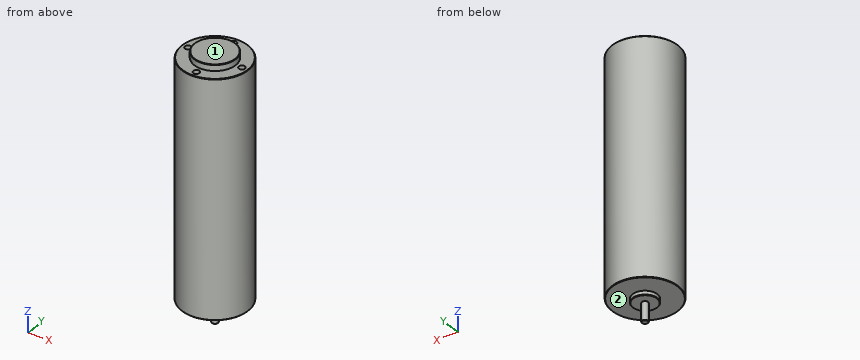
from build123d import *

# Parameters (mm, degrees)
CROQUIS1_R              = 16
SALIENTE_EXTRUIR1_DEPTH = 113.4
CROQUIS2_R              = 10
SALIENTE_EXTRUIR2_DEPTH = 3
CROQUIS3_R              = 6
SALIENTE_EXTRUIR3_DEPTH = 2
CROQUIS4_R              = 1.5
SALIENTE_EXTRUIR4_DEPTH = 9
CHAFL_N1_SIZE           = 0.2
CROQUIS5_R              = 1.5
CORTAR_EXTRUIR1_DEPTH   = 4


with BuildPart() as part:
    # Croquis1 → Saliente-Extruir1 (new body)
    with BuildSketch(Plane.XY):
        with Locations(Location((0, 0, 0), (0, 0, 180))):
            Circle(CROQUIS1_R)
    extrude(amount=SALIENTE_EXTRUIR1_DEPTH)

    # Croquis2 → Saliente-Extruir2 (add)
    with BuildSketch(Plane.XY.offset(113.4)):
        Circle(CROQUIS2_R)
    extrude(amount=SALIENTE_EXTRUIR2_DEPTH)

    # Croquis3 → Saliente-Extruir3 (add)
    with BuildSketch(Plane(origin=(0, 0, 0), x_dir=(-1, 0, 0), z_dir=(0, 0, -1))):
        Circle(CROQUIS3_R)
    extrude(amount=SALIENTE_EXTRUIR3_DEPTH)

    # Croquis4 → Saliente-Extruir4 (add)
    with BuildSketch(Plane(origin=(0, 0, -2), x_dir=(-1, 0, 0), z_dir=(0, 0, -1))):
        Circle(CROQUIS4_R)
    extrude(amount=SALIENTE_EXTRUIR4_DEPTH)

    # Chaflán1
    chafl_n1_edges = [part.edges().sort_by_distance(p)[0] for p in [
        (6, 0, -2),
        (1.5, 0, -11),
        (16, 0, 0),
        (16, 0, 113.4),
        (-10, 0, 116.4),
    ]]
    chamfer(chafl_n1_edges, length=CHAFL_N1_SIZE)

    # Croquis5 → Cortar-Extruir1 (cut)
    with BuildSketch(Plane.XY.offset(113.4)):
        with Locations((0, 13)):
            Circle(CROQUIS5_R)
        with Locations((13, 0)):
            Circle(CROQUIS5_R)
        with Locations((0, -13)):
            Circle(CROQUIS5_R)
        with Locations((-13, 0)):
            Circle(CROQUIS5_R)
    extrude(amount=-CORTAR_EXTRUIR1_DEPTH, mode=Mode.SUBTRACT)


solid = part.part
Can you work these out from the model? Positions are in its coordinate system, mm. Face numbers are marked on the shaded views. A direction names the side the tool comes from. Coordinates: 2 decimals unless noted, no trailing zeros. Loops run counter-clockwise (first coordinate to the right, second up) from the corner with the lowest first, then second, coordinate; pieces in that order, holes last. Notation, with made-up numbers: (-3.5, 72.5) - (23.5, 72.5) arc R16 cw to (23.5, 92.5) - close; hole circle Ø3 at (16.25, -28). An arc over 180 degrees is marked (long way). Put each result on its own line as item: value. Start each with the question number.
Item 1: If I drill on line 1 along Y through (x, z) = (0, 111); line 2 along Z through (x, y) = (12.5, -9); line 3 along Z through (x, y) = (5.5, -4), over which ranges is the centre line in solid material (lowest first)?
Item 2: For pin 1 (10 mm diameter, centred on x = 11, z = 16.5, fed in from -Y); pin 2 (2 mm diameter, centred on x = -4, y = -7.5, fed in from -Z); pin 3 (3 mm diameter, centred on y = 6.5, z = 36.5, fed in from +X), each with a flat end and sliding along its axis, tell me the tip position at first contact or that it passes through.
Item 3: Suppose I cut it at C-C (z = 95.5). Please give me the cut outline in (x, y), and give its area (3 significant figures).
Item 4: Which directions (+Z, -Z, +X, -X, +Y, -Y) give clear straight access to the entire face, cutting with the end or side of a thin tool? Please do the marked faces 1 and 2.
Here are the results:
1. line 1: -16 to -14.5, -11.5 to 11.5, 14.5 to 16
1. line 2: 0 to 113.4
1. line 3: 0 to 116.4
2. pin 1: y = -14.83
2. pin 2: z = 0
2. pin 3: x = 15.2
3. outline: circle Ø32 at (0, 0)
3. area: 804 mm²
4. face 1: +Z, +X, -X, +Y, -Y
4. face 2: -Z
